Here's how the part is built. I have some questions about the finished solid (model axes, mm). Round coordinates to 2 decimals unless told otherwise and drop trailing zeros. Order: outer loops, then holes, each group sorted by start corner. A loop starts at its lowest first (then second) coordinate and runs counter-clockwise, first axis right, second up.
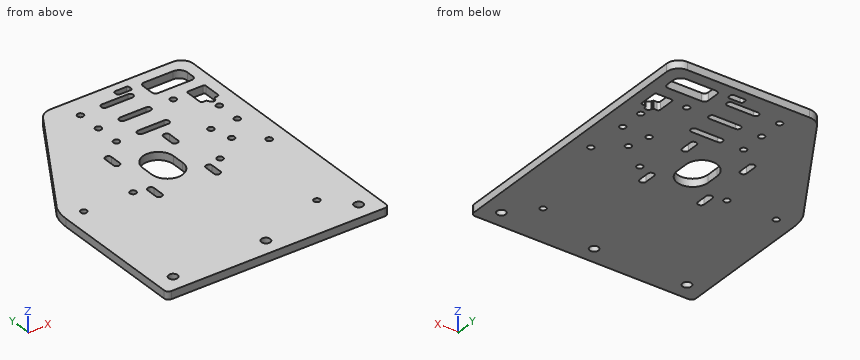
```python
from build123d import *

# Parameters (mm, degrees)
MODEL_R             = 3.5687
MODEL_R_2           = 2.50063
BOSS_EXTRUDE1_DEPTH = 6.35


with BuildPart() as part:
    # Model → Boss-Extrude1 (new body)
    with BuildSketch(Plane.XY):
        with BuildLine():
            Line((-195.531291458, -109.717656077), (-195.531291458, -0.364458494))
            ThreePointArc((-195.531291458, -0.364458494), (-194.811220192, 6.804036519), (-192.679778414, 13.686098661))
            Line((-192.679778414, 13.686098661), (-134.587886802, 108.667860444))
            ThreePointArc((-134.587886802, 108.667860444), (-130.212488604, 112.876263711), (-124.338469082, 114.409450622))
            Line((-124.338469082, 114.409450622), (-25.155306777, 114.409450622))
            ThreePointArc((-25.155306777, 114.409450622), (-18.320721917, 111.578459049), (-15.489778233, 104.743854352))
            Line((-15.489778233, 104.743854352), (-15.491291459, -109.717656077))
            ThreePointArc((-15.491291459, -109.717656077), (-16.476227854, -112.095502881), (-18.854074658, -113.080439277))
            Line((-18.854074658, -113.080439277), (-192.168508258, -113.080439277))
            ThreePointArc((-192.168508258, -113.080439277), (-194.546355062, -112.095502881), (-195.531291458, -109.717656077))
        make_face()
        with Locations((-105.511291458, -99.416633634)):
            Circle(MODEL_R, mode=Mode.SUBTRACT)
        with Locations((-30.191291459, -99.416633634)):
            Circle(MODEL_R, mode=Mode.SUBTRACT)
        with Locations((-180.831291458, -99.416633634)):
            Circle(MODEL_R, mode=Mode.SUBTRACT)
        with Locations((-112.800535337, 96.904216384)):
            Circle(MODEL_R_2, mode=Mode.SUBTRACT)
        with Locations((-112.800535337, 76.904216384)):
            Circle(MODEL_R_2, mode=Mode.SUBTRACT)
        with Locations((-112.800535337, 56.874490518)):
            Circle(MODEL_R_2, mode=Mode.SUBTRACT)
        with Locations((-52.065695289, 76.858190171)):
            Circle(MODEL_R_2, mode=Mode.SUBTRACT)
        with Locations((-53.581703018, 32.899307373)):
            Circle(MODEL_R_2, mode=Mode.SUBTRACT)
        with Locations((-49.191291458, 15.951915647)):
            Circle(MODEL_R_2, mode=Mode.SUBTRACT)
        with Locations((-32.191291412, 52.89930739)):
            Circle(MODEL_R_2, mode=Mode.SUBTRACT)
        with Locations((-32.191291073, 32.899307373)):
            Circle(MODEL_R_2, mode=Mode.SUBTRACT)
        with Locations((-30.23652443, 0.163856763)):
            Circle(MODEL_R_2, mode=Mode.SUBTRACT)
        with Locations((-70.191291459, -0.055133214)):
            Circle(MODEL_R_2, mode=Mode.SUBTRACT)
        with Locations((-140.831291458, -0.055133214)):
            Circle(MODEL_R_2, mode=Mode.SUBTRACT)
        with Locations((-180.831291459, -0.055133212)):
            Circle(MODEL_R_2, mode=Mode.SUBTRACT)
        with Locations((-49.191291458, -79.0480842)):
            Circle(MODEL_R_2, mode=Mode.SUBTRACT)
        with BuildLine():
            Line((-93.44346941, 94.43343728), (-72.443335776, 94.43343728))
            ThreePointArc((-72.443335776, 94.43343728), (-69.943334966, 96.93343809), (-72.443335776, 99.4334389))
            Line((-72.443335776, 99.4334389), (-93.44346941, 99.4334389))
            ThreePointArc((-93.44346941, 99.4334389), (-95.943470221, 96.93343809), (-93.44346941, 94.43343728))
        make_face(mode=Mode.SUBTRACT)
        with BuildLine():
            Line((-79.379374317, -12.874388322), (-79.379374317, -3.874412101))
            ThreePointArc((-79.379374317, -3.874412101), (-81.919367317, -1.334419101), (-84.459360317, -3.874412101))
            Line((-84.459360317, -3.874412101), (-84.459360317, -12.874388322))
            ThreePointArc((-84.459360317, -12.874388322), (-81.919367317, -15.414381322), (-79.379374317, -12.874388322))
        make_face(mode=Mode.SUBTRACT)
        with BuildLine():
            Line((-79.379374317, 34.36948148), (-79.379374317, 43.369457701))
            ThreePointArc((-79.379374317, 43.369457701), (-81.919367317, 45.909450701), (-84.459360317, 43.369457701))
            Line((-84.459360317, 43.369457701), (-84.459360317, 34.36948148))
            ThreePointArc((-84.459360317, 34.36948148), (-81.919367317, 31.82948848), (-79.379374317, 34.36948148))
        make_face(mode=Mode.SUBTRACT)
        with BuildLine():
            Line((-76.774493611, 102.430359236), (-67.894578253, 102.444637455))
            ThreePointArc((-67.894578253, 102.444637455), (-66.878577292, 102.865478833), (-66.457735914, 103.881479794))
            Line((-66.457735914, 103.881479794), (-66.457735914, 105.999769505))
            ThreePointArc((-66.457735914, 105.999769505), (-66.878577292, 107.015770466), (-67.894578253, 107.436611843))
            Line((-67.894578253, 107.436611843), (-76.992337138, 107.436611843))
            ThreePointArc((-76.992337138, 107.436611843), (-78.008338099, 107.015770466), (-78.429179476, 105.999769505))
            Line((-78.429179476, 105.999769505), (-78.443457695, 104.09932332))
            ThreePointArc((-78.443457695, 104.09932332), (-77.955415692, 102.918401239), (-76.774493611, 102.430359236))
        make_face(mode=Mode.SUBTRACT)
        with BuildLine():
            Line((-38.022285247, 62.781522119), (-35.552306408, 62.78308177))
            Line((-35.552306408, 62.78308177), (-34.582327568, 61.569828187))
            ThreePointArc((-34.582327568, 61.569828187), (-32.081364805, 59.175785763), (-29.582327568, 61.571838091))
            Line((-29.582327568, 61.571838091), (-28.612348728, 62.792230783))
            Line((-28.612348728, 62.792230783), (-26.426638777, 62.795800338))
            ThreePointArc((-26.426638777, 62.795800338), (-25.404720412, 63.283848845), (-24.989838628, 64.337595301))
            Line((-24.989838628, 64.337595301), (-24.989838628, 77.586949943))
            ThreePointArc((-24.989838628, 77.586949943), (-25.410680005, 78.602950904), (-26.426680966, 79.023792281))
            Line((-26.426680966, 79.023792281), (-38.022327436, 79.0380705))
            ThreePointArc((-38.022327436, 79.0380705), (-39.195708618, 78.575783886), (-39.685435446, 77.413587713))
            Line((-39.685435446, 77.413587713), (-39.69129152, 64.555438828))
            ThreePointArc((-39.69129152, 64.555438828), (-39.240439702, 63.307518511), (-38.022285247, 62.781522119))
        make_face(mode=Mode.SUBTRACT)
        with BuildLine():
            Line((-55.353814173, 88.936612327), (-28.125863081, 88.936612327))
            ThreePointArc((-28.125863081, 88.936612327), (-25.908358924, 89.855132624), (-24.989838628, 92.072636781))
            Line((-24.989838628, 92.072636781), (-24.989838628, 98.260334755))
            ThreePointArc((-24.989838628, 98.260334755), (-26.937319576, 102.961969673), (-31.638954494, 104.909450622))
            Line((-31.638954494, 104.909450622), (-55.353814173, 104.909450622))
            ThreePointArc((-55.353814173, 104.909450622), (-57.571318331, 103.990930325), (-58.489838627, 101.773426168))
            Line((-58.489838627, 101.773426168), (-58.489838627, 92.072636781))
            ThreePointArc((-58.489838627, 92.072636781), (-57.571318331, 89.855132624), (-55.353814173, 88.936612327))
        make_face(mode=Mode.SUBTRACT)
        with BuildLine():
            Line((-93.44346941, 74.433418373), (-72.443335776, 74.433418373))
            ThreePointArc((-72.443335776, 74.433418373), (-69.943334966, 76.933419183), (-72.443335776, 79.433419993))
            Line((-72.443335776, 79.433419993), (-93.44346941, 79.433419993))
            ThreePointArc((-93.44346941, 79.433419993), (-95.943470221, 76.933419183), (-93.44346941, 74.433418373))
        make_face(mode=Mode.SUBTRACT)
        with BuildLine():
            Line((-93.44346941, 54.43348809), (-72.443335776, 54.43348809))
            ThreePointArc((-72.443335776, 54.43348809), (-69.943347665, 56.9334762), (-72.443335776, 59.433464311))
            Line((-72.443335776, 59.433464311), (-93.44346941, 59.433464311))
            ThreePointArc((-93.44346941, 59.433464311), (-95.943457521, 56.9334762), (-93.44346941, 54.43348809))
        make_face(mode=Mode.SUBTRACT)
        with BuildLine():
            Line((-118.031293904, 10.239724211), (-118.031293904, 20.239724509))
            ThreePointArc((-118.031293904, 20.239724509), (-105.531294274, 32.73972451), (-93.031293902, 20.239725251))
            Line((-93.031293902, 20.239725251), (-93.031293902, 10.239724953))
            ThreePointArc((-93.031293902, 10.239724953), (-105.531293532, -2.260275048), (-118.031293904, 10.239724211))
        make_face(mode=Mode.SUBTRACT)
        with BuildLine():
            Line((-126.603228231, 43.369457701), (-126.603228231, 34.36948148))
            ThreePointArc((-126.603228231, 34.36948148), (-129.143221232, 31.82948848), (-131.683214232, 34.36948148))
            Line((-131.683214232, 34.36948148), (-131.683214232, 43.369457701))
            ThreePointArc((-131.683214232, 43.369457701), (-129.143221232, 45.909450701), (-126.603228231, 43.369457701))
        make_face(mode=Mode.SUBTRACT)
        with BuildLine():
            Line((-131.683214232, -12.874388322), (-131.683214232, -3.874412101))
            ThreePointArc((-131.683214232, -3.874412101), (-129.143221232, -1.334419101), (-126.603228231, -3.874412101))
            Line((-126.603228231, -3.874412101), (-126.603228231, -12.874388322))
            ThreePointArc((-126.603228231, -12.874388322), (-129.143221232, -15.414381322), (-131.683214232, -12.874388322))
        make_face(mode=Mode.SUBTRACT)
    extrude(amount=BOSS_EXTRUDE1_DEPTH)


solid = part.part
```
1. If we section it at A-A, the plane y = 72: Write out the boundary of the cut face in (x, z).
Evaluation:
outline: (-157.01, 0) - (-39.69, 0) - (-39.69, 6.35) - (-157.01, 6.35) - close; (-24.99, 0) - (-15.49, 0) - (-15.49, 6.35) - (-24.99, 6.35) - close
2. I need wall thicknesses on probe 1 along X at (y, z) = (-6, 6); probe 2 along Y at (x, z) = (-76.5, 5.25); probe 3 along Y at (x, z) = (-28, 4.5). Which ranges of each line are inside material? Lowest first, please.
Evaluation:
probe 1: x = -195.53 to -131.68, -126.6 to -84.46, -79.38 to -15.49
probe 2: y = -113.08 to 54.43, 59.43 to 74.43, 79.43 to 94.43, 99.43 to 102.43, 107.44 to 114.41
probe 3: y = -113.08 to -102.23, -96.6 to -0.95, 1.28 to 62.79, 79.03 to 88.94, 103.83 to 114.41
3. I'm going to push flat-ended pins straight in: P1, Ø1.9, axis at y = 17, z = 3, coming from the -X side; P2, Ø3, axis at y = 37, z = 4.5, coming from the -X side. Where does each tip first touch, or does it pass through?
Evaluation:
P1: stops at x = -191.23
P2: stops at x = -179.34
4. If we section it at B-B, the plane x = -147.5: Write out the boundary of the cut face in (y, z).
Evaluation:
outline: (-113.08, 0) - (87.56, 0) - (87.56, 6.35) - (-113.08, 6.35) - close
5. If we section it at C-C, the plane z = 1.25: State how many separate pieces and enclosed holes the cut face has, and give its area (3 significant figures).
Evaluation:
separate pieces: 1
enclosed holes: 27
area: 34,900 mm2
